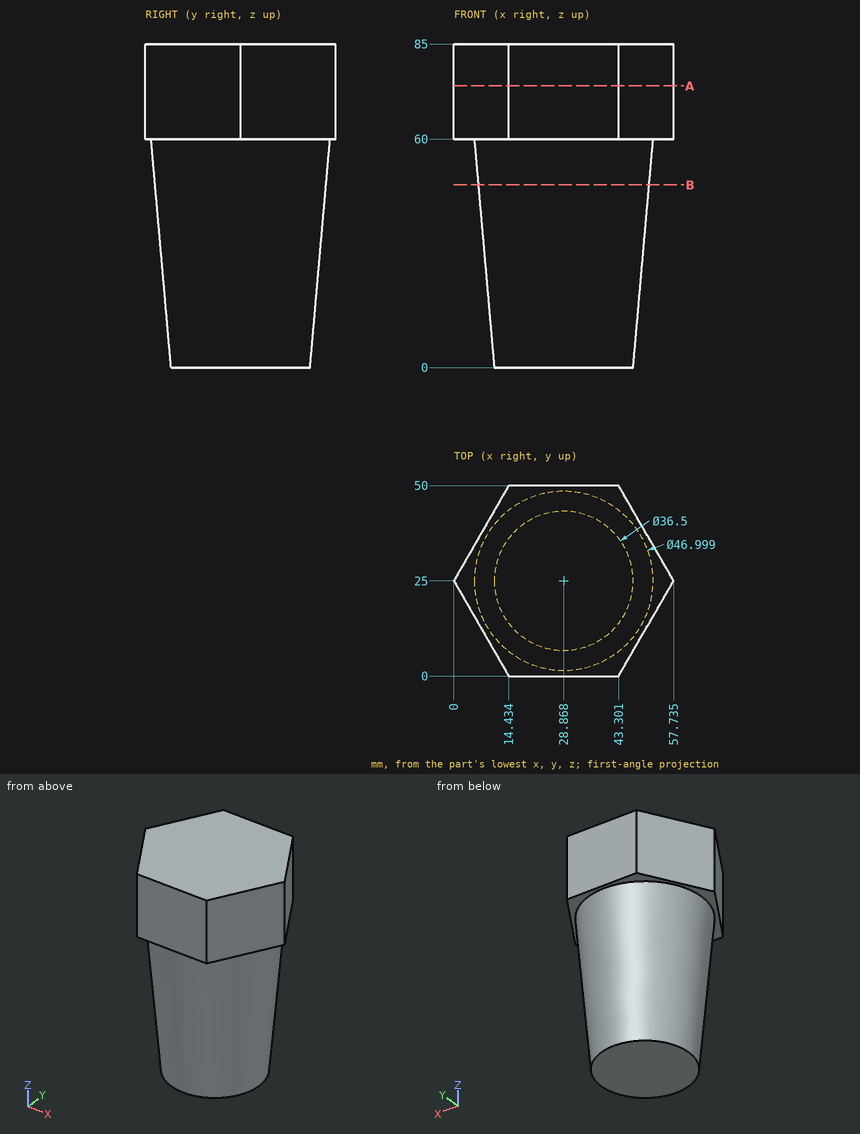
Study the drawing (mm; zero at the part's minimum x, y, z) and answer. Round coordinates to 2 decimals unless told otherwise and drop trailing zeros. Loops run counter-clockwise (first coordinate to the right, second up) from the corner with the lowest first, then second, coordinate; pieces in that order, holes last. Notation, with made-up numbers: (18.5, 76.5) -> (64.5, 76.5) arc R12 cw to (64.5, 84.5) -> close; hole circle Ø7 at (48.25, 85). An arc over 180 degrees is marked (long way). One line per item, written item: value.
1) A cutting plane is placed at B-B (z = 48). Determine the outline of the cut face in (x, y).
Answer list:
outline: circle Ø44.9 at (28.87, 25)
2) A cutting plane is placed at A-A (z = 74). Determine the outline of the cut face in (x, y) (1 decimal).
Answer list:
outline: (0, 25) -> (14.4, 0) -> (43.3, 0) -> (57.7, 25) -> (43.3, 50) -> (14.4, 50) -> close
3) Flat-ended cylindrical pins translate along their axes: P1, Ø5, axis at x = 48, y = 5, coming from the +Z side; P2, Ø6, axis at x = 27, z = 34.5, coming from the -Y side; P3, Ø1.5, axis at x = 23.5, z = 18.5, coming from the +Y side; P4, Ø1.5, axis at y = 24, z = 69.5, coming from the -X side (1 decimal). Find the tip coordinate at first contact, or state that the pin passes through.
Answer list:
P1: stops at z = 85
P2: stops at y = 3.5
P3: stops at y = 44.34
P4: stops at x = 0.1
4) Consider L1, parallel to Z at x = 46, y = 44; L2, parallel to Y at x = 23.5, z = 54; L3, parallel to Y at x = 43, z = 40.5. Determine where each line is inside the solid, lowest interval first. Write a range as [from, to].
Answer list:
L1: z = [60, 85]
L2: y = [2.66, 47.34]
L3: y = [8.41, 41.59]
